Geometry: final body of the model. Coordinates: model frame, mm. A direction names the side the tool comes from. Coordinates: 2 decimals unless noted, no trailing zeros. Order: outer loops, then holes, each group sorted by start corner. A loop starts at its lowest first (then second) coordinate and runs counter-clockwise, first axis right, second up. Notation, with made-up numbers: (-12, -26) - (-4, -26) arc R27 cw to (-4, -1) - close; hole circle Ø9 at (-14, -20.75). An arc over 180 degrees is marked (long way). Use a Markdown table: item, result. Add a question column.
Autodesk Inventor part; units mm, degrees
ref_plane "YZ Plane" through (0, 0, 0) normal (1, 0, 0) x (0, 1, 0)
ref_plane "XZ Plane" through (0, 0, 0) normal (0, 1, 0) x (-1, 0, 0)
ref_plane "XY Plane" through (0, 0, 0) normal (0, 0, 1) x (1, 0, 0)
sketch "Sketch1" plane through (0, 0, 0) normal (1, 0, 0) x (0, 1, 0)
  line L0 (-254, 203.2) -> (254, 203.2)
  line L1 (254, 203.2) -> (254, -203.2)
  line L2 (254, -203.2) -> (-254, -203.2)
  line L3 (-254, -203.2) -> (-254, 203.2)
  line L4 (-254, 203.2) -> (254, -203.2) construction
  line L5 (254, 203.2) -> (-254, -203.2) construction
  point P0 (0, 0)
  dimension "d0" = 406.4
  dimension "d1" = 508
extrude "Extrusion1" add sketch "Sketch1" along normal mid plane 12.7
sketch "Sketch2" plane through (6.35, 0, 0) normal (1, 0, 0) x (0, 0, -1)
  circle A0 centre (-63.5, -203.2) radius 5
  line L0 (203.2, -254) -> (203.2, 254)
  line L1 (203.2, 254) -> (-203.2, 254)
  line L2 (-203.2, 254) -> (-203.2, -254)
  line L3 (-203.2, -254) -> (203.2, -254)
  circle A1 centre (63.5, -203.2) radius 5
  circle A2 centre (-63.5, -152.4) radius 5
  circle A3 centre (63.5, -152.4) radius 5
  point P0 (0, 0)
  dimension "d6" = 127
  dimension "d9" = 50.8
  dimension "d12" = 10
  dimension "d14" = 63.5
  dimension "d15" = 50.8
extrude "Extrusion2" cut sketch "Sketch2" against normal blind 12.7 contours A0 | A1 | A2 | A3
sketch "Sketch3" plane through (-6.35, -254, 203.2) normal (0, 0, 1) x (1, 0, 0)
  line L0 (0, 508) -> (12.7, 508)
  line L1 (12.7, 0) -> (12.7, 508)
  line L2 (0, 508) -> (12.7, 508)
  line L3 (12.7, 508) -> (12.7, 254)
  line L4 (12.7, 254) -> (0, 254)
  line L5 (0, 254) -> (0, 508)
  point P0 (6.35, 254)
  dimension "d26" = 254
extrude "Extrusion3" add sketch "Sketch3" along normal blind 50.8
sketch "Sketch4" plane through (6.35, 0, 0) normal (1, 0, 0) x (0, 0, -1)
  line L0 (-254, 157.8) -> (-203.2, 157.8)
  line L1 (-203.2, 157.8) -> (-203.2, 72)
  line L2 (-203.2, 72) -> (-254, 72)
  line L3 (-254, 72) -> (-254, 157.8)
  line L4 (-254, 0) -> (-254, 254)
  line L5 (203.2, 254) -> (-254, 254)
  point P0 (0, 0)
  dimension "d20" = 0
  dimension "d21" = 96.2
  dimension "d22" = 50.8
  dimension "d23" = 85.8
extrude "Extrusion4" cut sketch "Sketch4" against normal blind 50.8
properties part number "Wood-6"
1) Draft query along Y for faces 4 (the flat face through (-6.35, -4, 22)), 5 (the flat face through (0, 254, 22)), 6 (the flat face through (0, 116, 203.2)). Return one class per face: released by +Y, released by -Y, zero draft, split by the parting line, or undercut.
2) Line query: line 1 (Y direction, x = -1.5, z = -63.5); line 2 (Y direction, x = 5, z = 218); line 3 (Y direction, x = -5.5, z = -65). Output: solid intervals per line, ascending. Write a range as from..to.
3) First-contact query: pin 1 (9 mm diameter, centred on y = -152.4, z = -63.5, fed in from -X); pin 2 (1.5 mm diameter, centred on x = 2.5, y = -105.5, fed in from +Z); pin 3 (16 mm diameter, centred on y = -203.2, z = -63.5, fed in from -X). Flat tips, straight axial feed; report the tip coordinate or a pass-through.
4) Access query for faces 1 (the flat face through (0, 4, -203.2)), 2 (the flat face through (0, 72, 228)), 3 (the flat face through (0, -129, 203.2)). Directions: +Z, -Z, +X, -X, +Y, -Y. A direction counts if a zero-diameter tool reaches every point of the face in a straight line with its end or side. Return the directions, or none.
5) Section query B-B (y = 113). Return the cut outline in (x, z), and give its area (3 significant figures).
6) Section query A-A (x = -2.25). Return the cut outline in (y, z), and give its area (3 significant figures).
From the geometry:
| question | item | result |
|---|---|---|
| 1 | face 4 | zero draft |
| 1 | face 5 | released by +Y |
| 1 | face 6 | undercut |
| 2 | line 1 | y = -254..-208.2, -198.2..-157.4, -147.4..254 |
| 2 | line 2 | y = 0..72, 157.8..254 |
| 2 | line 3 | y = -254..-207.97, -198.43..-157.17, -147.63..254 |
| 3 | pin 1 | passes through |
| 3 | pin 2 | stops at z = 203.2 |
| 3 | pin 3 | stops at x = -6.35 |
| 4 | face 1 | -Z, +X, -X, +Y, -Y |
| 4 | face 2 | +Z, +X, -X |
| 4 | face 3 | +Z, +X, -X, -Y |
| 5 | outline | (-6.35, -203.2) - (6.35, -203.2) - (6.35, 203.2) - (-6.35, 203.2) - close |
| 5 | area | 5,160 mm^2 |
| 6 | outline | (-254, -203.2) - (254, -203.2) - (254, 254) - (157.8, 254) - (157.8, 203.2) - (72, 203.2) - (72, 254) - (0, 254) - (0, 203.2) - (-254, 203.2) - close; hole circle Ø10 at (-203.2, -63.5); hole circle Ø10 at (-203.2, 63.5); hole circle Ø10 at (-152.4, -63.5); hole circle Ø10 at (-152.4, 63.5) |
| 6 | area | 215,000 mm^2 |
